from build123d import *

# Parameters (mm, degrees)
F0_R     = 31.75
F0_R_2   = 28.575
F1_DEPTH = 304.8
F2_W     = 6.35
F2_H     = 28.575
F3_DEPTH = 25.4
F6_DEPTH = 165.1
F7_W     = 19.05
F7_H     = 19.05
F7_W_2   = 12.7
F7_H_2   = 12.7


# Not quite as in the source:
# - a feature names something its author has since deleted; it is built from what else it names


with BuildPart() as f1:
    # F0 (on Top) → F1 (new body)
    with BuildSketch(Plane.XY):
        Circle(F0_R)
        Circle(F0_R_2, mode=Mode.SUBTRACT)
    extrude(amount=-F1_DEPTH)

    # F2 (on Top) → F3 (join)
    with BuildSketch(Plane.XY):
        with Locations((0, -42.8625)):
            Rectangle(F2_W, F2_H)
    extrude(amount=-F3_DEPTH)

    # F5 (on offset) → F6 (join)
    with BuildSketch(Plane.XZ.offset(-76.2)):
        Polygon((-76.2, 0), (76.2, 0), (76.2, 44.45), (69.85, 44.45), (69.85, 6.35), (-69.85, 6.35), (-69.85, 44.45), (-76.2, 44.45), align=None)
    extrude(amount=F6_DEPTH)

    # F9: sweep along a path in F8
    with BuildLine(Plane.XY.offset(6.35)) as f9_path:
        Line((98.425, 76.2), (98.425, -917.575))
        Line((98.425, -917.575), (76.2, -939.8))
        Line((76.2, -939.8), (-76.2, -939.8))
        Line((-76.2, -939.8), (-98.425, -917.575))
        Line((-98.425, -917.575), (-98.425, 76.2))
    # F7 (on offset) → F9 (sweep)
    with BuildSketch(Plane.XZ.offset(-76.2)):
        with Locations((85.725, 9.525)):
            Rectangle(F7_W, F7_H)
        with Locations((85.725, 9.525)):
            Rectangle(F7_W_2, F7_H_2, mode=Mode.SUBTRACT)
    sweep(path=f9_path.line, transition=Transition.RIGHT)


solid = f1.part
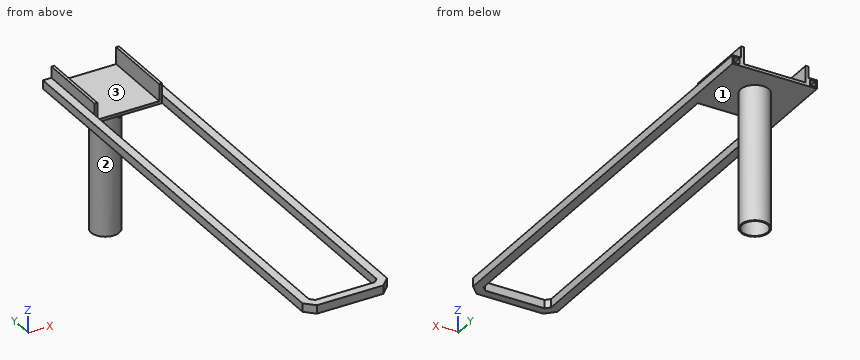
Verification items for the finished model (mm, model axes). Face numbers are marked on the shaded views. Give positions to 0.01 mm unless a question says otherwise; leave off trailing zeros. Write each loop counter-clockwise with the first axis right and the second up, starting at its lowest first coordinate (ties: lowest second). Pieces come first, ordered by that corner, then holes. Notation, with made-up numbers: (26, -34) - (47, -34) arc R31 ccw to (47, -7) - close; hole circle Ø7 at (5, -21). An arc over 180 degrees is marked (long way). Answer as CSV lines item,"result". Start each with the question number.
1. Sectioned sample at B-B (x = 43). Record the boundary of the cut face in (y, z) (3 decimals), then the cut area to 3 significant figures.
2. Sectioned sample at A-A (y = -256.5). Record the boundary of the cut face in (x, z) (3 decimals).
3. Thickness scan on line 1 (Y direction, x = 0, z = -144) (3 decimals); line 2 (Z direction, x = -86.5, y = 27) (3 decimals). Record the ranges inside material, lowest first.
4. Sectioned sample at D-D (z = -246). Record the boundary of the cut face in (x, y) (3 decimals), then the cut area to 3 significant figures.
5. Sectioned sample at C-C (y = 0). Record the boundary of the cut face in (x, z) (3 decimals).
6. Depth check by flat-ended pin: pin 1 (5 mm diameter, centred on y = -35.5, z = -182.5, fed in from +X); pin 2 (7.5 mm diameter, centred on y = -35.5, z = 34, fed in from -X); pin 3 (1.9 mm diameter, centred on x = 1, y = -45, fed in from -Z); pin 4 (10 mm diameter, centred on x = -2, z = -97, fed in from -Y). Enter the tip coordinate at first touch or a pass-through.
7. Draft check along X on the marked faces 1, 2 and 3. Enter one of: pulls with the +X half, pulls with the -X half, needs draft (parallel to the pull), parting line crosses it, or undercut.
Derived:
1,outline,"(-936.625, 0) - (-917.575, 0) - (-917.575, 19.05) - (-936.625, 19.05) - close; (-88.9, 0) - (76.2, 0) - (76.2, 6.35) - (-88.9, 6.35) - close; hole (-933.45, 3.175) - (-920.75, 3.175) - (-920.75, 15.875) - (-933.45, 15.875) - close"
1,area,"1,250 mm²"
2,outline,"(-95.25, 0) - (-76.2, 0) - (-76.2, 19.05) - (-95.25, 19.05) - close; (76.2, 0) - (95.25, 0) - (95.25, 19.05) - (76.2, 19.05) - close; hole (-92.075, 3.175) - (-79.375, 3.175) - (-79.375, 15.875) - (-92.075, 15.875) - close; hole (79.375, 3.175) - (92.075, 3.175) - (92.075, 15.875) - (79.375, 15.875) - close"
3,line 1,"-31.75 to -28.575, 28.575 to 31.75"
3,line 2,"0 to 3.175, 15.875 to 19.05"
4,outline,"circle Ø63.5 at (0, 0); hole circle Ø57.15 at (0, 0)"
4,area,"602 mm²"
5,outline,"(-95.25, 0) - (-31.75, 0) - (-31.75, -304.8) - (-28.575, -304.8) - (-28.575, 0) - (28.575, 0) - (28.575, -304.8) - (31.75, -304.8) - (31.75, 0) - (95.25, 0) - (95.25, 19.05) - (76.2, 19.05) - (76.2, 44.45) - (69.85, 44.45) - (69.85, 6.35) - (-69.85, 6.35) - (-69.85, 44.45) - (-76.2, 44.45) - (-76.2, 19.05) - (-95.25, 19.05) - close; hole (-92.075, 3.175) - (-79.375, 3.175) - (-79.375, 15.875) - (-92.075, 15.875) - close; hole (79.375, 3.175) - (92.075, 3.175) - (92.075, 15.875) - (79.375, 15.875) - close"
6,pin 1,"through"
6,pin 2,"x = -76.2"
6,pin 3,"z = -25.4"
6,pin 4,"y = -31.75"
7,face 1,"needs draft"
7,face 2,"parting line crosses it"
7,face 3,"undercut"
